Input: part model. Units: mm. Frame: model coordinates. Face numbers are marked on the shaded views. A direction names the side the tool comes from. Give positions to 0.01 mm unless a question says otherwise; leave off trailing zeros. Order: outer loops, then holes, each group sorted by start corner. A loop starts at its lowest first (then second) coordinate and runs counter-clockwise, first axis right, second up. Notation, with made-up numbers: M -4.5,70 L 34.5,70 A22 ccw 34.5,86 Z; hole C 13,-9.5 d11. An arc over 180 degrees is marked long. Use a Markdown table: item, result.
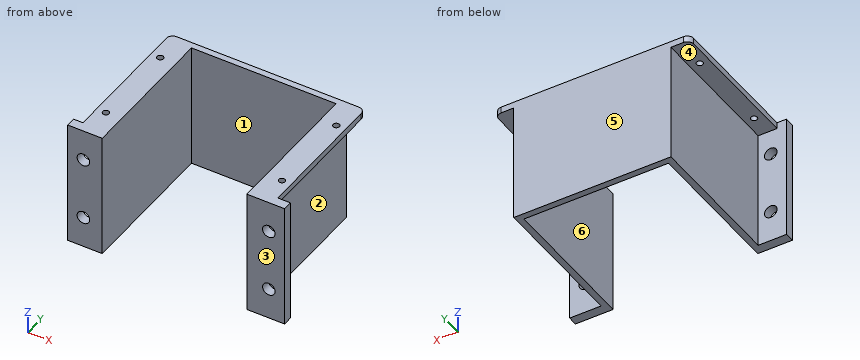
from build123d import *

# Parameters (mm, degrees)
SKETCH012_W      = 10
SKETCH012_H      = 40
SKETCH012_R      = 2
EXTRUDE010_DEPTH = 3
EXTRUDE008_DEPTH = 40
SKETCH011_W      = 6
SKETCH011_H      = 48
SKETCH011_R      = 1
EXTRUDE009_DEPTH = 2
FILLET002_R      = 2


with BuildPart() as extrude010:
    # Sketch012 → Extrude010 (new body)
    with BuildSketch(Plane.XZ):
        with Locations((-9, -18)):
            Rectangle(SKETCH012_W, SKETCH012_H)
        with Locations((-9, -8)):
            Circle(SKETCH012_R, mode=Mode.SUBTRACT)
        with Locations((-9, -28)):
            Circle(SKETCH012_R, mode=Mode.SUBTRACT)
        with Locations((50, -18)):
            Rectangle(SKETCH012_W, SKETCH012_H)
        with Locations((50, -8)):
            Circle(SKETCH012_R, mode=Mode.SUBTRACT)
        with Locations((50, -28)):
            Circle(SKETCH012_R, mode=Mode.SUBTRACT)
    extrude(amount=EXTRUDE010_DEPTH)


with BuildPart() as extrude008:
    # Sketch007 → Extrude008 (new body)
    with BuildSketch(Plane.XY.offset(2)):
        Polygon((43, -3), (43, 43), (-3, 43), (-3, -3), (-5, -3), (-5, 45), (45, 45), (45, -3), align=None)
    extrude(amount=-EXTRUDE008_DEPTH)


with BuildPart() as fusion006:
    # Sketch011 → Extrude009 (new body)
    with BuildSketch(Plane.XY.offset(2)):
        with Locations((48, 21)):
            Rectangle(SKETCH011_W, SKETCH011_H)
        with Locations((48, 35)):
            Circle(SKETCH011_R, mode=Mode.SUBTRACT)
        with Locations((48, 7)):
            Circle(SKETCH011_R, mode=Mode.SUBTRACT)
        with Locations((-8, 21)):
            Rectangle(SKETCH011_W, SKETCH011_H)
        with Locations((-8, 7)):
            Circle(SKETCH011_R, mode=Mode.SUBTRACT)
        with Locations((-8, 35)):
            Circle(SKETCH011_R, mode=Mode.SUBTRACT)
    extrude(amount=-EXTRUDE009_DEPTH)

    # Fillet002
    fillet002_edges = [fusion006.edges().sort_by_distance(p)[0] for p in [
        (-11, 45, 1),
        (51, 45, 1),
    ]]
    fillet(fillet002_edges, radius=FILLET002_R)

    # Fusion005: union Extrude008
    add(extrude008.part)

    # Fusion006: union Extrude010
    add(extrude010.part)


solid = fusion006.part
1) Cut plane B-B on y = 7. Return loops of the section in (x, z), and give its area (3 significant figures).
Response values:
| item | result |
|---|---|
| outline | M -11,0 L -9,0 L -9,2 L -11,2 Z; M -7,0 L -5,0 L -5,-38 L -3,-38 L -3,2 L -7,2 Z; M 43,-38 L 45,-38 L 45,0 L 47,0 L 47,2 L 43,2 Z; M 49,0 L 51,0 L 51,2 L 49,2 Z |
| area | 176 mm² |
2) Material intervals for line 1 (Z direction, x = 50, y = -2.15); line 2 (Y direction, x = 48, z = 1.3); line 3 (X direction, y = 27, z = -6.5), sorted ascending. Write a range as from..to.
Response values:
| item | result |
|---|---|
| line 1 | z = -38..-30, -26..-10, -6..2 |
| line 2 | y = -3..6, 8..34, 36..45 |
| line 3 | x = -5..-3, 43..45 |
3) Cut plane A-A on y = 2. Return loops of the section in (x, z).
Response values:
| item | result |
|---|---|
| outline | M -11,0 L -5,0 L -5,-38 L -3,-38 L -3,2 L -11,2 Z; M 43,-38 L 45,-38 L 45,0 L 51,0 L 51,2 L 43,2 Z |
4) Cut plane C-C on z = -18. Return loops of the section in (x, y).
Response values:
| item | result |
|---|---|
| outline | M -14,-3 L -3,-3 L -3,43 L 43,43 L 43,-3 L 55,-3 L 55,0 L 45,0 L 45,45 L -5,45 L -5,0 L -14,0 Z |
5) First-contact query: pin 1 Ø2.5 at (x, y) = (-8, 7) entering from -Z; pin 2 Ø8 at (y, z) = (36, -14.5) entering from -X; pin 3 Ø6.5 at (x, z) = (-9, -8) entering from +Y. Flat tips, straight axial feed; report the tip coordinate or a pass-through.
Response values:
| item | result |
|---|---|
| pin 1 | stops at z = 0 |
| pin 2 | stops at x = -5 |
| pin 3 | stops at y = 0 |
6) Cut plane D-D on x = -8. Return loops of the section in (y, z), and give its area (3 significant figures).
Response values:
| item | result |
|---|---|
| outline | M -3,-38 L 0,-38 L 0,-29.73 L -3,-29.73 Z; M -3,-26.27 L 0,-26.27 L 0,-9.73 L -3,-9.73 Z; M -3,-6.27 L 0,-6.27 L 0,0 L 6,0 L 6,2 L -3,2 Z; M 8,0 L 34,0 L 34,2 L 8,2 Z; M 36,0 L 45,0 L 45,2 L 36,2 Z |
| area | 181 mm² |
7) Reachability of the marked faces 4, 5 and 6 from +Z, -Z, +X, -X, +Y, -Y: full face, straight path, thin tool, end or side. Return the list, or none.
Response values:
| item | result |
|---|---|
| face 4 | -Z, -X, +Y |
| face 5 | +Z, -Z, +X, -X, +Y |
| face 6 | +Z, -Z, -Y |
8) Mould query, pull axis X, two halves, no side actions, for the marked faces 1, 2 and 3. Classes: released by +X, released by -X, zero draft, split by the parting line, or undercut.
Response values:
| item | result |
|---|---|
| face 1 | undercut |
| face 2 | released by +X |
| face 3 | zero draft |
